Design review of the part shown in the three views and the two pictorial views. Dimensions are in mm from the part's minimum x, y and z. A direction names the side the tool comes from. Give positions to 0.01 mm unless a question says otherwise; leave off trailing zeros. Loops run counter-clockwise (first coordinate to the right, second up) from the corner with the lowest first, then second, coordinate; pieces in that order, holes last.
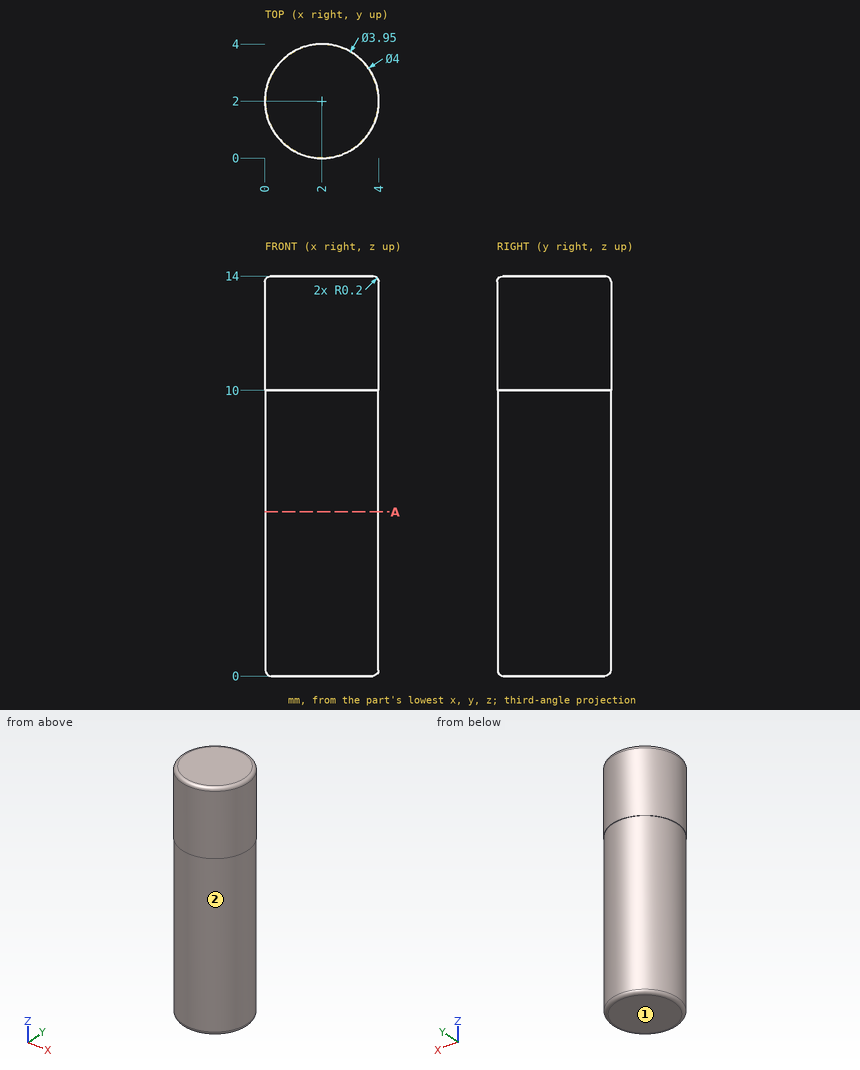
Q1. Machinability: for the marked faces 1 and 2, which of the approach directions +Z, -Z, +X, -X, +Y, -Y give a long, thin tool a straight path to every point of the face, cutting with its end or side? Answer none if there is none.
Answers:
face 1: -Z, +X, -X, +Y, -Y
face 2: -Z
Q2. For pin 1 Ø1.5 at (x, z) = (2.5, 8) entering from +Y (3 decimals); pin 2 Ø1.2 at (x, y) = (1, 3) entering from -Z, all flat-tipped, find the tip position at first contact; note any pin that passes through.
Answers:
pin 1: stops at y = 3.975
pin 2: stops at z = 0
Q3. Consider section A-A on z = 5.75. Give the boundary of the cut face in (x, y) (3 decimals), plus the area to 3 significant figures.
Answers:
outline: circle Ø3.95 at (2, 2)
area: 12.3 mm2
Q4. For probe 1 along Y at (x, z) = (1.9, 11.25); probe 2 along X at (y, z) = (1.6, 4.75); probe 3 along X at (y, z) = (2.1, 5.5), list the stretches that pass through material, from the lowest coordinate up.
Answers:
probe 1: y = 0 to 4
probe 2: x = 0.07 to 3.93
probe 3: x = 0.03 to 3.97
